from build123d import *

# Parameters (mm, degrees)
SKETCH3_W                = 30
SKETCH3_H                = 39.99999999999999
SKETCH3_R                = 2.2500000000000107
BOSS_EXTRUDE1_DEPTH      = 5
BOSS_EXTRUDE2_DEPTH      = 7
BOSS_EXTRUDE2_DEPTH_BACK = 7
BOSS_EXTRUDE3_DEPTH      = 4.493237048
BOSS_EXTRUDE4_DEPTH      = 2
BOSS_EXTRUDE5_DEPTH      = 10
SKETCH8_R                = 0.874999999999402
SKETCH8_R_2              = 0.8749999999993996
CUT_EXTRUDE1_DEPTH       = 128.20148900625736
CHAMFER1_SIZE            = 16.49


with BuildPart() as part:
    # Sketch3 → Boss-Extrude1 (new body)
    with BuildSketch(Plane(origin=(-20.656096268089573, 72.16840410421906, 1.396e-13), x_dir=(0.9613952185534441, 0.2751712807372447, 0), z_dir=(0.2751712807372447, -0.9613952185534441, -1.905836610257915e-15))):
        with Locations((81.70857094012555, -8.293237047851846)):
            Rectangle(SKETCH3_W, SKETCH3_H)
        with Locations((92.70857094012555, 7.706762952148144)):
            Circle(SKETCH3_R, mode=Mode.SUBTRACT)
        with Locations((70.70857094012555, 7.706762952148144)):
            Circle(SKETCH3_R, mode=Mode.SUBTRACT)
        with Locations((92.70857094012555, -24.293237047851843)):
            Circle(SKETCH3_R, mode=Mode.SUBTRACT)
        with Locations((70.70857094012555, -24.293237047851843)):
            Circle(SKETCH3_R, mode=Mode.SUBTRACT)
    extrude(amount=BOSS_EXTRUDE1_DEPTH)

    # Sketch4 → Boss-Extrude2 (add, two sides: drawn at the far end of the back side and taken through both)
    with BuildSketch(Plane.XY.offset(-8.293237047851855).offset(-BOSS_EXTRUDE2_DEPTH_BACK)):
        with BuildLine():
            Line((73.69491783056992, 93.97284933531479), (44.8530612739666, 85.71771091319745))
            Line((44.8530612739666, 85.71771091319745), (21.868275221764016, 30.766725890030358))
            ThreePointArc((21.868275221764016, 30.766725890030358), (24.444464826602115, 21.20831351558636), (34.00287720104611, 23.78450312042446))
            Line((34.00287720104611, 23.78450312042446), (73.69491783056992, 93.97284933531479))
        make_face()
    extrude(amount=BOSS_EXTRUDE2_DEPTH + BOSS_EXTRUDE2_DEPTH_BACK)

    # Sketch5 → Boss-Extrude3 (add)
    with BuildSketch(Plane.XY.offset(-1.2932370478518544)):
        with BuildLine():
            Line((34.00287720104611, 23.78450312042448), (39.63747674144046, 33.74829477867678))
            Line((39.63747674144046, 33.74829477867678), (26.275931115955906, 41.30434988526449))
            Line((26.275931115955906, 41.30434988526449), (21.868275221764016, 30.766725890030376))
            ThreePointArc((21.868275221764016, 30.766725890030376), (24.444464826602115, 21.20831351558638), (34.00287720104611, 23.78450312042448))
        make_face()
    extrude(amount=BOSS_EXTRUDE3_DEPTH)

    # Sketch6 → Boss-Extrude4 (add)
    with BuildSketch(Plane.XY.offset(3.199999999999975)):
        with BuildLine():
            Line((14.367137951998398, 12.833346791724153), (22.10488555177782, 16.08852481695844))
            ThreePointArc((22.10488555177782, 16.08852481695844), (23.553783162359977, 19.026709419920138), (20.85003386751253, 20.876566927309664))
            Line((20.85003386751253, 20.876566927309664), (17.573963093227494, 20.50007903397223))
            Line((17.573963093227494, 20.50007903397223), (26.275931115955906, 41.30434988526449))
            Line((26.275931115955906, 41.30434988526449), (39.63747674144046, 33.74829477867678))
            Line((39.63747674144046, 33.74829477867678), (27.851332502459574, 12.906585477167601))
            Line((27.851332502459574, 12.906585477167601), (18.71941105293458, 10.372103436249658))
            Line((18.71941105293458, 10.372103436249658), (14.367137951998398, 12.833346791724153))
        make_face()
    extrude(amount=BOSS_EXTRUDE4_DEPTH)

    # Sketch9 → Boss-Extrude5 (add)
    with BuildSketch(Plane.XY.offset(5.199999999999974)):
        Polygon((19.512348726132714, 25.134283574349986), (26.275931115955906, 41.30434988526451), (39.637476741440466, 33.74829477867679), (27.851332502459464, 12.906585477167425), (18.719411052934504, 10.37210343624943), (14.367137951998316, 12.833346791723917), (11.755774091436686, 14.310092805008848), (15.614590337202541, 23.53557583742582), align=None)
    extrude(amount=BOSS_EXTRUDE5_DEPTH)

    # Sketch8 → Cut-Extrude1 (cut, through all)
    with BuildSketch(Plane.XY.offset(3.199999999999975)):
        with Locations((21.135456701762944, 18.39291360897205)):
            Circle(SKETCH8_R)
        with Locations((16.298803780568512, 17.12532198707588)):
            Circle(SKETCH8_R_2)
    extrude(amount=CUT_EXTRUDE1_DEPTH, mode=Mode.SUBTRACT)

    # Chamfer1
    chamfer1_edges = [part.edges().sort_by_distance(p)[0] for p in [
        (32.95670392869818, 37.52632233197063, -1.2932370478518544),
    ]]
    chamfer(chamfer1_edges, length=CHAMFER1_SIZE)


solid = part.part
Verification items for the finished model (mm, model axes). A direction names the side the tool comes from. Give positions to 0.01 mm unless a question says otherwise; leave off trailing zeros. Write each loop counter-clockwise with the first axis right and the second up, starting at its lowest first coordinate (ties: lowest second). Pieces come first, ordered by that corner, then holes. Notation, with made-up numbers: (26.5, 52.5) - (81.5, 52.5) arc R16 ccw to (81.5, 64.5) - close; hole circle Ø3 at (9.5, -6.5). An arc over 180 degrees is marked (long way). Answer as CSV lines item,"result". Start each with the question number.
1. Sectioned sample at C-C (z = -19). Record the boundary of the cut face in (x, y).
2. Depth check by flat-ended pin: pin 1 (20.5 mm diameter, centred on x = 43, y = 81, fed in from +Z); pin 2 (20.5 mm diameter, centred on x = 24, y = 18, fed in from -Z); pin 3 (10 mm diameter, centred on x = 37.5, y = 53, fed in from +Z). Enter the tip coordinate at first touch or a pass-through.
3. Sectioned sample at B-B (y = 50). Record the boundary of the cut face in (x, z).
4. Draft check along X on faces 5 (the face through (58, 92, 11.707)), 6 (the face through (24.31, 21.29, -6.18)), 7 (the face through (47.719, 89.175, -22.062)), 8 (the face through (46.284, 88.764, 6.338)). Enter one of: pulls with the +X half, pulls with the -X half, needs draft (parallel to the pull), parting line crosses it, or undercut.
5. Sectioned sample at D-D (z = -4.5). Record the boundary of the cut face in (x, y), then the cut area to 3 significant figures.
6. Set-up check for faces 1 (the face through (44.156, 88.155, -8.573)), 2 (the face through (17.536, 24.324, 10.13)), 3 (the face through (18.182, 14.438, 4.186)), 4 (the face through (23.566, 18.978, 4.186)): record each of +Z, -Z, +X, -X, +Y, -Y from which the full face is reachable in a straight line by a thin tool's end or side.
7. Thickness scan on line 1 (Z direction, x = 65.5, y = 95.5); line 2 (Z direction, x = 48.5, y = 61); line 3 (Y direction, x = 23, z = -11). Record the ranges inside material, lowest first.
Derived:
1,outline,"(43.48, 90.52) - (44.85, 85.72) - (73.69, 93.97) - (72.32, 98.78) - close"
2,pin 1,"z = 11.71"
2,pin 2,"z = -15.29"
2,pin 3,"z = 4.49"
3,outline,"(29.91, -15.29) - (48.83, -15.29) - (48.83, -1.29) - (44.4, -1.29) - (29.91, 5.84) - close"
4,face 5,"needs draft"
4,face 6,"parting line crosses it"
4,face 7,"undercut"
4,face 8,"undercut"
5,outline,"(21.87, 30.77) arc R7 ccw to (34, 23.78) - (73.69, 93.97) - (72.32, 98.78) - (43.48, 90.52) - (44.85, 85.72) - close"
5,area,"1,490 mm²"
6,face 1,"+Z, -Z, -X"
6,face 2,"+Z, -Z, -X, +Y"
6,face 3,"-Z, -X"
6,face 4,"-Z"
7,line 1,"-28.29 to 11.71"
7,line 2,"-15.29 to -1.29"
7,line 3,"22.31 to 33.47"
